from build123d import *

# Parameters (mm, degrees)
CROQUIS2_R              = 1.85
CROQUIS2_R_2            = 10
CROQUIS2_R_3            = 11
SALIENTE_EXTRUIR1_DEPTH = 21.5
CROQUIS3_W              = 13.5
CROQUIS3_H              = 13.5
CORTAR_EXTRUIR1_DEPTH   = 227.063412752
MATRIZC1_COUNT          = 6
SALIENTE_EXTRUIR2_START = -4
CROQUIS4_R              = 11
CROQUIS4_R_2            = 5.5
SALIENTE_EXTRUIR2_DEPTH = 4
CORTAR_EXTRUIR2_START   = -10
CROQUIS5_R              = 1.6
CROQUIS5_R_2            = 5.5
CORTAR_EXTRUIR2_DEPTH   = 10


with BuildPart() as part:
    # Croquis2 → Saliente-Extruir1 (new body)
    with BuildSketch(Plane(origin=(0, 0, 0), x_dir=(1, 0, 0), z_dir=(0, 1, 0))):
        with BuildLine():
            Line((34.338474425, 90.387328615), (65.023396068, 71.560868943))
            Line((65.023396068, 71.560868943), (57.99870039, 46.557847845))
            ThreePointArc((57.99870039, 46.557847845), (57.540985683, 39.344606317), (60.071411753, 32.574281363))
            ThreePointArc((60.071411753, 32.574281363), (64.365061572, 26.760080874), (70.66006642, 23.20856429))
            Line((70.66006642, 23.20856429), (95.446959973, 15.455673128))
            Line((95.446959973, 15.455673128), (94.485228455, -20.531478364))
            Line((94.485228455, -20.531478364), (69.319629174, -26.949424002))
            ThreePointArc((69.319629174, -26.949424002), (62.843921414, -30.159652201), (58.245861047, -35.736227938))
            ThreePointArc((58.245861047, -35.736227938), (55.357440631, -42.361738001), (55.42923947, -49.589130408))
            Line((55.42923947, -49.589130408), (61.108485548, -74.931655487))
            Line((61.108485548, -74.931655487), (29.461832387, -92.092347306))
            Line((29.461832387, -92.092347306), (11.320928784, -73.507271847))
            ThreePointArc((11.320928784, -73.507271847), (5.302935731, -69.504258519), (-1.825550706, -68.310509301))
            ThreePointArc((-1.825550706, -68.310509301), (-9.007620942, -69.121818875), (-15.23082695, -72.797694698))
            Line((-15.23082695, -72.797694698), (-34.338474425, -90.387328615))
            Line((-34.338474425, -90.387328615), (-65.023396068, -71.560868943))
            Line((-65.023396068, -71.560868943), (-57.99870039, -46.557847845))
            ThreePointArc((-57.99870039, -46.557847845), (-57.540985683, -39.344606317), (-60.071411753, -32.574281363))
            ThreePointArc((-60.071411753, -32.574281363), (-64.365061572, -26.760080874), (-70.66006642, -23.20856429))
            Line((-70.66006642, -23.20856429), (-95.446959973, -15.455673128))
            Line((-95.446959973, -15.455673128), (-94.485228455, 20.531478364))
            Line((-94.485228455, 20.531478364), (-69.319629174, 26.949424002))
            ThreePointArc((-69.319629174, 26.949424002), (-62.843921414, 30.159652201), (-58.245861047, 35.736227938))
            ThreePointArc((-58.245861047, 35.736227938), (-55.357440631, 42.361738001), (-55.42923947, 49.589130408))
            Line((-55.42923947, 49.589130408), (-61.108485548, 74.931655487))
            Line((-61.108485548, 74.931655487), (-29.461832387, 92.092347306))
            Line((-29.461832387, 92.092347306), (-11.320928784, 73.507271847))
            ThreePointArc((-11.320928784, 73.507271847), (-5.302935731, 69.504258519), (1.825550706, 68.310509301))
            ThreePointArc((1.825550706, 68.310509301), (9.007620942, 69.121818875), (15.23082695, 72.797694698))
            Line((15.23082695, 72.797694698), (34.338474425, 90.387328615))
        make_face()
        with Locations(Location((45.497277541, 74.155227303, 0), (0, 0, 270))):
            Circle(CROQUIS2_R, mode=Mode.SUBTRACT)
        with Locations(Location((26.147860656, 42.617946726, 0), (0, 0, 270))):
            Circle(CROQUIS2_R, mode=Mode.SUBTRACT)
        with Locations(Location((36.084047705, 58.812766481, 0), (0, 0, 270))):
            Circle(CROQUIS2_R_2, mode=Mode.SUBTRACT)
        with Locations(Location((0, 0, 0), (0, 0, 270))):
            Circle(CROQUIS2_R, mode=Mode.SUBTRACT)
        with Locations(Location((43.953684946, 23.834294194, 0), (0, 0, 270))):
            Circle(CROQUIS2_R_3, mode=Mode.SUBTRACT)
        with Locations(Location((68.975373692, -1.843318743, 0), (0, 0, 270))):
            Circle(CROQUIS2_R_2, mode=Mode.SUBTRACT)
        with Locations(Location((86.968949438, -2.324184502, 0), (0, 0, 270))):
            Circle(CROQUIS2_R, mode=Mode.SUBTRACT)
        with Locations(Location((49.98215485, -1.33573822, 0), (0, 0, 270))):
            Circle(CROQUIS2_R, mode=Mode.SUBTRACT)
        with Locations(Location((42.617946726, -26.147860656, 0), (0, 0, 270))):
            Circle(CROQUIS2_R_3, mode=Mode.SUBTRACT)
        with Locations(Location((32.891325987, -60.656085225, 0), (0, 0, 270))):
            Circle(CROQUIS2_R_2, mode=Mode.SUBTRACT)
        with Locations(Location((41.471671897, -76.479411805, 0), (0, 0, 270))):
            Circle(CROQUIS2_R, mode=Mode.SUBTRACT)
        with Locations(Location((23.834294194, -43.953684946, 0), (0, 0, 270))):
            Circle(CROQUIS2_R, mode=Mode.SUBTRACT)
        with Locations(Location((-1.33573822, -49.98215485, 0), (0, 0, 270))):
            Circle(CROQUIS2_R_3, mode=Mode.SUBTRACT)
        with Locations(Location((-36.084047705, -58.812766481, 0), (0, 0, 270))):
            Circle(CROQUIS2_R_2, mode=Mode.SUBTRACT)
        with Locations(Location((-45.497277541, -74.155227303, 0), (0, 0, 270))):
            Circle(CROQUIS2_R, mode=Mode.SUBTRACT)
        with Locations(Location((-26.147860656, -42.617946726, 0), (0, 0, 270))):
            Circle(CROQUIS2_R, mode=Mode.SUBTRACT)
        with Locations(Location((-43.953684946, -23.834294194, 0), (0, 0, 270))):
            Circle(CROQUIS2_R_3, mode=Mode.SUBTRACT)
        with Locations(Location((-68.975373692, 1.843318743, 0), (0, 0, 270))):
            Circle(CROQUIS2_R_2, mode=Mode.SUBTRACT)
        with Locations(Location((-86.968949438, 2.324184502, 0), (0, 0, 270))):
            Circle(CROQUIS2_R, mode=Mode.SUBTRACT)
        with Locations(Location((-49.98215485, 1.33573822, 0), (0, 0, 270))):
            Circle(CROQUIS2_R, mode=Mode.SUBTRACT)
        with Locations(Location((-42.617946726, 26.147860656, 0), (0, 0, 270))):
            Circle(CROQUIS2_R_3, mode=Mode.SUBTRACT)
        with Locations(Location((-32.891325987, 60.656085225, 0), (0, 0, 270))):
            Circle(CROQUIS2_R_2, mode=Mode.SUBTRACT)
        with Locations(Location((-41.471671897, 76.479411805, 0), (0, 0, 270))):
            Circle(CROQUIS2_R, mode=Mode.SUBTRACT)
        with Locations(Location((-23.834294194, 43.953684946, 0), (0, 0, 270))):
            Circle(CROQUIS2_R, mode=Mode.SUBTRACT)
        with Locations(Location((1.33573822, 49.98215485, 0), (0, 0, 270))):
            Circle(CROQUIS2_R_3, mode=Mode.SUBTRACT)
    extrude(amount=SALIENTE_EXTRUIR1_DEPTH)

    # Croquis3 → Cortar-Extruir1 (cut, through all)
    with BuildSketch(Plane(origin=(45.285158968, 0, 83.512001397), x_dir=(0.8790736989108549, 0, -0.4766858838723754), z_dir=(0.4766858838723755, 0, 0.879073698910855))):
        with Locations((0, 10.75)):
            Rectangle(CROQUIS3_W, CROQUIS3_H)
    cortar_extruir1 = extrude(amount=-CORTAR_EXTRUIR1_DEPTH, mode=Mode.SUBTRACT)

    # MatrizC1: Cortar-Extruir1 ×6 about axis
    matrizc1_axis = Axis((0, 0, 0), (0, 1, 0))
    for i in range(1, MATRIZC1_COUNT):
        add(cortar_extruir1.rotate(matrizc1_axis, i * 360 / MATRIZC1_COUNT), mode=Mode.SUBTRACT)

    # Croquis4 → Saliente-Extruir2 (add)
    with BuildSketch(Plane(origin=(0, 21.5, 0), x_dir=(1, 0, 0), z_dir=(0, 1, 0)).offset(SALIENTE_EXTRUIR2_START)):
        with Locations(Location((-42.617946726, 26.147860656, 0), (0, 0, 270))):
            Circle(CROQUIS4_R)
        with Locations(Location((-42.617946726, 26.147860656, 0), (0, 0, 270))):
            Circle(CROQUIS4_R_2, mode=Mode.SUBTRACT)
    extrude(amount=SALIENTE_EXTRUIR2_DEPTH)

    # Croquis5 → Cortar-Extruir2 (cut)
    with BuildSketch(Plane(origin=(0, 21.5, 0), x_dir=(1, 0, 0), z_dir=(0, 1, 0)).offset(CORTAR_EXTRUIR2_START)):
        with Locations(Location((-47.056631996, 42.558164525, 0), (0, 0, 270))):
            Circle(CROQUIS5_R)
        with Locations(Location((-42.617946726, 26.147860656, 0), (0, 0, 270))):
            Circle(CROQUIS5_R_2)
        with Locations(Location((-26.207642857, 30.586545927, 0), (0, 0, 270))):
            Circle(CROQUIS5_R)
        with Locations(Location((-38.179261455, 9.737556787, 0), (0, 0, 270))):
            Circle(CROQUIS5_R)
        with Locations(Location((-59.028250595, 21.709175385, 0), (0, 0, 270))):
            Circle(CROQUIS5_R)
    extrude(amount=CORTAR_EXTRUIR2_DEPTH, mode=Mode.SUBTRACT)


solid = part.part
Input: part model. Units: mm. Frame: model coordinates. A direction names the side the tool comes from. Give positions to 0.01 mm unless a question says otherwise; leave off trailing zeros. Loops run counter-clockwise (first coordinate to the right, second up) from the corner with the lowest first, then second, coordinate; pieces in that order, holes last. Notation, with made-up numbers: (-37.75, -22.75) -> (6.25, -22.75) arc R10 ccw to (6.25, -3.75) -> close; hole circle Ø8 at (86.25, 32.5). An arc over 180 degrees is marked (long way). Answer as a JSON object with one key per item and string values. Group by question number.
Item 1: Pin query (flat end, axial travel): P1, Ø2.5, axis at x = -59.03, z = -21.71, coming from the +Y side; P2, Ø10, axis at y = 12.5, z = -15, coming from the -X side; P3, Ø1.5, axis at x = -6.5, y = 17.5, coming from the +Z side; P4, Ø4.5, axis at x = 23.83, z = 43.95, coming from the -Y side. Return the tip coordinate at first contact, or that it passes through.
Item 2: Pull-direction query (Y, two-part tool) for faces 4 (the flat face through (1, 21.5, 19)), 5 (the flat face through (11.707, 10.656, 35.749)), 6 (the flat face through (-34.85, 10.66, -78.43)), 7 (the cylindrical face through (5.398, 10.599, 69.542)); classes: released by +Y, released by -Y, zero draft, split by the parting line, or undercut.
Item 3: Cut plane A-A, the plane x = -4.5. Return the cut outline in (y, z), and give its area (3 significant figures).
Item 4: Cut plane B-B, the plane y = 8. State how many separate pieces and enclosed holes the cut face has, and give its area (3 significant figures).
Item 5: Line query: probe 1 along Z at (x, y) = (7, 17); probe 2 along Z at (x, y) = (5, 7.25); probe 3 along Y at (x, z) = (3, 15). Output: solid intervals per line, ascending.
Item 6: Reachability of faces 1 (the cylindrical face through (-64.289, 10.599, 26.828)), 2 (the cylindrical face through (-5.398, 10.599, -69.542)), 3 (the flat face through (-23.24, 10.66, -28.7)) from +Z, -Z, +X, -X, +Y, -Y: full face, straight path, thin tool, end or side. Return the list, or none.
Checks:
{
 "1": {"P1": "stops at y = 11.5", "P2": "stops at x = -94.77", "P3": "stops at z = 68.63", "P4": "stops at y = 0"},
 "2": {"face 4": "released by +Y", "face 5": "undercut", "face 6": "undercut", "face 7": "zero draft"},
 "3": {"outline": "(0, -69.21) -> (21.5, -69.21) -> (21.5, -59.31) -> (0, -59.31) -> close; (0, -40.66) -> (21.5, -40.66) -> (21.5, 39.45) -> (0, 39.45) -> close; (0, 60.52) -> (21.5, 60.52) -> (21.5, 68.26) -> (0, 68.26) -> close; hole (4, -22.46) -> (17.5, -22.46) -> (17.5, 20.24) -> (4, 20.24) -> close", "area": "1,530 mm²"},
 "4": {"separate pieces": "6", "enclosed holes": "6", "area": "12,400 mm²"},
 "5": {"probe 1": "z = -68.58 to -59.41, -40.55 to -24.32, 27.07 to 42.8, 57.16 to 70.28", "probe 2": "z = -68.29 to -60.35, -39.61 to -21.06, 23.38 to 40.99, 58.97 to 69.39", "probe 3": "y = 0 to 4, 17.5 to 21.5"},
 "6": {"face 1": "-X, +Y, -Y", "face 2": "-Z, +Y, -Y", "face 3": "none"}
}
